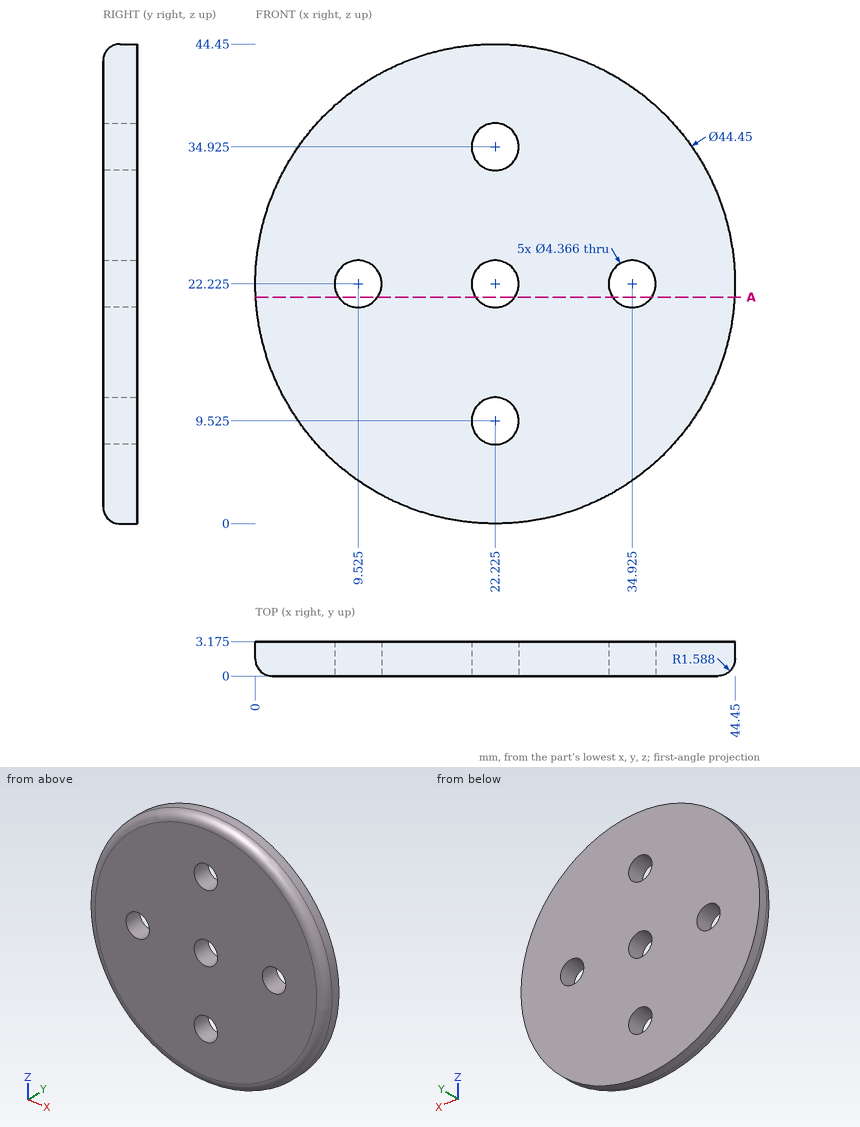
Input: dimensioned drawing with shaded views. Units: mm. Origin: part minimum x, y, z. Round coordinates to 2 decimals unless told otherwise and drop trailing zeros. Use one line per item in the form item = value. Start each with the question number.
1) First-contact query: P1, Ø5, axis at x = 22.225, z = 34.925, coming from the -Y side. Flat tip, straight axial feed; report the tip coordinate or a pass-through.
2) Line query: L1, parallel to Z at x = 21, y = 2.25 (1 decimal); L2, parallel to X at y = 2.2, z = 9 (1 decimal); L3, parallel to Z at x = 14, y = 1.6. Output: solid intervals per line, ascending.
3) Section A-A on z = 21. Give the number of separate pieces and of enclosed holes in the cut face.
Response:
q1.P1 = 0
q2.L1 = 0 to 7.7, 11.3 to 20.4, 24 to 33.1, 36.7 to 44.4
q2.L2 = 4.4 to 20.1, 24.3 to 40.1
q2.L3 = 1.58 to 42.87
q3.separate_pieces = 4
q3.enclosed_holes = 0
